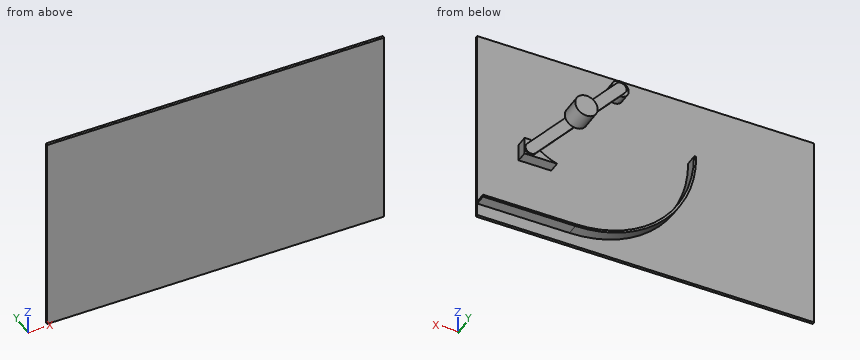
```python
from build123d import *

# Parameters (mm, degrees)
SKETCH1_W           = 1500
SKETCH1_H           = 900
BOSS_EXTRUDE1_DEPTH = 12
BOSS_EXTRUDE2_DEPTH = 50
BOSS_EXTRUDE3_DEPTH = 50
BOSS_EXTRUDE4_DEPTH = 6.35
SKETCH5_R           = 38.1
BOSS_EXTRUDE5_DEPTH = 50
SKETCH6_R           = 50
BOSS_EXTRUDE6_DEPTH = 90


with BuildPart() as part:
    # Sketch1 → Boss-Extrude1 (new body)
    with BuildSketch(Plane(origin=(0, 0, 0), x_dir=(1, 0, 0), z_dir=(0, 1, 0))):
        Rectangle(SKETCH1_W, SKETCH1_H)
    extrude(amount=BOSS_EXTRUDE1_DEPTH)

    # Sketch2 → Boss-Extrude2 (add)
    with BuildSketch(Plane(origin=(0, 12, 0), x_dir=(1, 0, 0), z_dir=(0, 1, 0))):
        with BuildLine():
            Line((339, 382.8), (750, 382.8))
            Line((750, 382.8), (750, 392.8))
            Line((750, 392.8), (339, 392.8))
            ThreePointArc((339, 392.8), (-41.423448278, 235.223448278), (-199, -145.2))
            ThreePointArc((-199, -145.2), (-194, -150.2), (-189, -145.2))
            ThreePointArc((-189, -145.2), (-34.352380466, 228.152380466), (339, 382.8))
        make_face()
    extrude(amount=BOSS_EXTRUDE2_DEPTH)

    # Sketch3 → Boss-Extrude3 (add)
    with BuildSketch(Plane(origin=(0, 12, 0), x_dir=(1, 0, 0), z_dir=(0, 1, 0))):
        with BuildLine():
            Line((564.991489323, 108.8), (420.319677815, 108.8))
            ThreePointArc((420.319677815, 108.8), (485.283321394, 77.802421247), (539.591489323, 30.561043498))
            Line((539.591489323, 30.561043498), (564.991489323, 30.561043498))
            Line((564.991489323, 30.561043498), (564.991489323, 108.8))
        make_face()
    extrude(amount=BOSS_EXTRUDE3_DEPTH)

    # Sketch4 → Boss-Extrude4 (add)
    with BuildSketch(Plane(origin=(0, 62, 0), x_dir=(1, 0, 0), z_dir=(0, 1, 0))):
        with BuildLine():
            Line((120.609259907, -352.445373029), (519.438207109, 95.812890558))
            ThreePointArc((519.438207109, 95.812890558), (555.298232366, 97.905398285), (557.390740093, 62.045373029))
            Line((557.390740093, 62.045373029), (158.561792891, -386.212890558))
            ThreePointArc((158.561792891, -386.212890558), (122.701767634, -388.305398285), (120.609259907, -352.445373029))
        make_face()
    extrude(amount=BOSS_EXTRUDE4_DEPTH)

    # Sketch5 → Boss-Extrude5 (add)
    with BuildSketch(Plane(origin=(0, 12, 0), x_dir=(1, 0, 0), z_dir=(0, 1, 0))):
        with Locations(Location((139.585526399, -369.329131794, 0), (0, 0, 90.149856959))):
            Circle(SKETCH5_R)
    extrude(amount=BOSS_EXTRUDE5_DEPTH)

    # Sketch6 → Boss-Extrude6 (add)
    with BuildSketch(Plane(origin=(0, 68.35, 0), x_dir=(1, 0, 0), z_dir=(0, 1, 0))):
        with Locations(Location((339, -145.2, 0), (0, 0, 78.870244402))):
            Circle(SKETCH6_R)
    extrude(amount=BOSS_EXTRUDE6_DEPTH)


solid = part.part
```
Design review of the part built by this model. Coordinates are the model's own, in mm. Give positions to 0.01 mm unless a question says otherwise; leave off trailing zeros. Write each loop counter-clockwise with the first axis right and the second up, starting at its lowest first coordinate (ties: lowest second). Pieces come first, ordered by that corner, then holes.
(1) Wall thickness on line 1 along Y through (x, z) = (684, 230); line 2 along Y through (x, z) = (115.5, 365.5); line 3 along Z through (x, y) = (604, 37.5): over which ranges is each line inside the solid? List them lowest first.
Checked values:
line 1: y = 0 to 12
line 2: y = 0 to 68.35
line 3: z = -392.8 to -382.8
(2) Clearance check with flat-ended pins moving along their axes: pin 1 Ø6 at (x, z) = (-381, -339.5) entering from +Y; pin 2 Ø23 at (x, z) = (150.5, 356) entering from +Y; pin 3 Ø1.5 at (y, z) = (64.5, 16) entering from +X. State where each tip first meets the part, or that it passes through.
Checked values:
pin 1: stops at y = 12
pin 2: stops at y = 68.35
pin 3: stops at x = 488.62
(3) Add section C-C (x = -294). Give the boundary of the cut face in (y, z), and give its area (3 significant figures).
Checked values:
outline: (0, -450) - (12, -450) - (12, 450) - (0, 450) - close
area: 10,800 mm2
(4) Add section B-B (z = -268.5). Give the boundary of the cut face in (x, y), and give its area (3 significant figures).
Checked values:
outline: (-750, 0) - (750, 0) - (750, 12) - (10.92, 12) - (10.92, 62) - (-4.94, 62) - (-4.94, 12) - (-750, 12) - close
area: 18,800 mm2
(5) Add section A-A (x = 448.5). Give the boundary of the cut face in (y, z).
Checked values:
outline: (0, -450) - (12, -450) - (12, -392.8) - (62, -392.8) - (62, -382.8) - (12, -382.8) - (12, -108.8) - (62, -108.8) - (62, -97.98) - (12, -97.98) - (12, 450) - (0, 450) - close; (62, -16.08) - (68.35, -16.08) - (68.35, 60.34) - (62, 60.34) - close
(6) Add section D-D (y = 90). Give the boundary of the cut face in (x, z), and give its area (3 significant figures).
Checked values:
outline: circle Ø100 at (339, 145.2)
area: 7,850 mm2
